Could you check a few things on this drawing? It's one solid part, dimensions in mm from its lowest x, y, z. Give positions to 0.01 mm unless a question says otherwise; leave off trailing zeros. Order: outer loops, then holes, each group sorted by start corner. A loop starts at its lowest first (then second) coordinate and runs counter-clockwise, first axis right, second up. Notation, with made-up numbers: (76, 38) - (135, 38) arc R22 cw to (135, 53) - close; hole circle Ø5 at (55.5, -37.5). An arc over 180 degrees is marked (long way). Put each result on its own line as item: value.
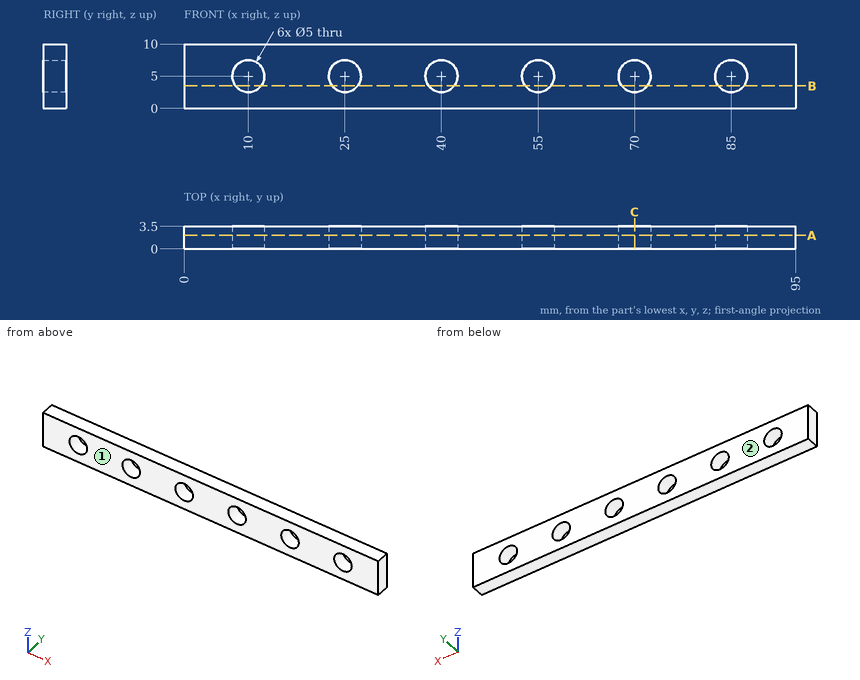
1) I'm going to push a flat-ended pin straight in: pin 1 (4 mm diameter, centred on x = 70, z = 5, fed in from +Y). Where does the tip first touch, or does it pass through?
Filled in:
pin 1: passes through
2) Suppose I cut it at A-A, the plane y = 2.1. List the corners of the cut face in (x, z) for me.
Filled in:
outline: (0, 0) - (95, 0) - (95, 10) - (0, 10) - close; hole circle Ø5 at (10, 5); hole circle Ø5 at (25, 5); hole circle Ø5 at (40, 5); hole circle Ø5 at (55, 5); hole circle Ø5 at (70, 5); hole circle Ø5 at (85, 5)
3) We'd pull the mould along Y, two halves only. Please class the marked faces 1 and 2: pulls with the +Y half, pulls with the -Y half, needs draft (parallel to the pull), parting line crosses it, or undercut.
Filled in:
face 1: pulls with the -Y half
face 2: pulls with the +Y half
4) Suppose I cut it at C-C, the plane x = 70. List the corners of the cut face in (y, z) for me.
Filled in:
outline: (0, 0) - (3.5, 0) - (3.5, 2.5) - (0, 2.5) - close; (0, 7.5) - (3.5, 7.5) - (3.5, 10) - (0, 10) - close
5) If I drill on line 1 (Z direction, x = 40, y = 2.7); line 2 (Z direction, x = 38, y = 2.15), over which ranges is the centre line in solid material (lowest first)? Write a range as [from, to].
Filled in:
line 1: z = [0, 2.5], [7.5, 10]
line 2: z = [0, 3.5], [6.5, 10]
6) Suppose I cut it at B-B, the plane z = 3.5. List the corners of the cut face in (x, y) for me, and give its area (4 significant figures).
Filled in:
outline: (0, 0) - (8, 0) - (8, 3.5) - (0, 3.5) - close; (12, 0) - (23, 0) - (23, 3.5) - (12, 3.5) - close; (27, 0) - (38, 0) - (38, 3.5) - (27, 3.5) - close; (42, 0) - (53, 0) - (53, 3.5) - (42, 3.5) - close; (57, 0) - (68, 0) - (68, 3.5) - (57, 3.5) - close; (72, 0) - (83, 0) - (83, 3.5) - (72, 3.5) - close; (87, 0) - (95, 0) - (95, 3.5) - (87, 3.5) - close
area: 248.5 mm^2
